from build123d import *

# Parameters (mm, degrees)
ESTRUSIONE_ESTRUSIONE1_DEPTH = 11
SCHIZZO4_R                   = 12
TAGLIO_ESTRUSIONE1_DEPTH     = 64.600314465
FORO_5_0_5_1_D               = 5
FORO_5_0_5_2_D               = 5
RACCORDO1_R                  = 0.2


with BuildPart() as part:
    # Schizzo2 → Estrusione-Estrusione1 (new body)
    with BuildSketch(Plane(origin=(0, 0, 0), x_dir=(1, 0, 0), z_dir=(0, 0, -1))):
        Polygon((-60, -8), (-60, 8), (-45, 8), (-45, 18), (45, 18), (45, 8), (60, 8), (60, -8), (45, -8), (45, -18), (-45, -18), (-45, -8), align=None)
    extrude(amount=-ESTRUSIONE_ESTRUSIONE1_DEPTH)

    # Schizzo4 → Taglio-Estrusione1 (cut, through all)
    with BuildSketch(Plane.XY.offset(11)):
        Circle(SCHIZZO4_R)
    extrude(amount=-TAGLIO_ESTRUSIONE1_DEPTH, mode=Mode.SUBTRACT)

    # Foro Ø5.0 (5)-1 (through all)
    with Locations(Plane(origin=(0, -18, 0), x_dir=(-1, 0, 0), z_dir=(0, -1, 0))):
        with Locations((0, -5.5)):
            Hole(FORO_5_0_5_1_D / 2)

    # Foro Ø5.0 (5)-2 (through all)
    with Locations(Plane.XY.offset(11)):
        with Locations((-52.5, 0), (52.5, 0)):
            Hole(FORO_5_0_5_2_D / 2)

    # Raccordo1
    raccordo1_edges = [part.edges().sort_by_distance(p)[0] for p in [
        (45, -8, 5.5),
        (45, 8, 5.5),
        (-45, 8, 5.5),
        (-45, -8, 5.5),
    ]]
    fillet(raccordo1_edges, radius=RACCORDO1_R)


solid = part.part
Source: CAD feature listing. Evaluate the final solid. Frame: model axes, mm. A direction names the side the tool comes from. Give positions to 0.01 mm unless a question says otherwise; leave off trailing zeros. Loops run counter-clockwise (first coordinate to the right, second up) from the corner with the lowest first, then second, coordinate; pieces in that order, holes last. Notation, with made-up numbers: (34, 10) -> (85, 10) arc R9 cw to (85, 24) -> close; hole circle Ø4 at (68.5, 21.25). An arc over 180 degrees is marked (long way). Use a Markdown table: item, result. Add a question column.
1) Reachability of faces 4 (the face through (-53, -8, 5)), 5 (the face through (-52, 8, 5)), 6 (the face through (53, 8, 5)), 7 (the face through (52, -8, 5)) from +Z, -Z, +X, -X, +Y, -Y: full face, straight path, thin tool, end or side. Return the list, or none.
2) Section query A-A, the plane y = 0. Return the cut outline in (x, z).
3) Section query B-B, the plane x = -52.5. Return the cut outline in (y, z), then the cut area to 3 significant figures.
4) Section query D-D, the plane x = 0. Return the cut outline in (y, z), then the cut area to 3 significant figures.
5) First-contact query: pin 1 (5 mm diameter, centred on y = -12, z = 8, fed in from +X); pin 2 (5 mm diameter, centred on y = 13, z = 4.5, fed in from -X); pin 3 (1 mm diameter, centred on x = -47.5, z = 2, fed in from -Y). Flat tips, straight axial feed; report the tip coordinate or a pass-through.
6) Line query: line 1 along Z through (x, y) = (0, 13.5); line 2 along Y through (x, z) = (0, 2.5); line 3 along Y through (x, z) = (-52.5, 7.25). Output: solid intervals per line, ascending. Write a range as [from, to].
7) Section query C-C, the plane z = 1.5. Return the cut outline in (x, y), then the cut area to 3 significant figures.
8) Pull-direction query (X, two-part tool) for faces 1 (the face through (50.19, -0.96, 5.42)), 2 (the face through (-45, 13, 5)), 3 (the face through (0.8, -12.3, 11)); classes: +X half, -X half, draft (parallel to the pull), parting line (faces both ways), or undercut.
Numbers:
| question | item | result |
|---|---|---|
| 1 | face 4 | +Z, -Z, -X, -Y |
| 1 | face 5 | +Z, -Z, -X, +Y |
| 1 | face 6 | +Z, -Z, +X, +Y |
| 1 | face 7 | +Z, -Z, +X, -Y |
| 2 | outline | (-60, 0) -> (-55, 0) -> (-55, 11) -> (-60, 11) -> close; (-50, 0) -> (-12, 0) -> (-12, 11) -> (-50, 11) -> close; (12, 0) -> (50, 0) -> (50, 11) -> (12, 11) -> close; (55, 0) -> (60, 0) -> (60, 11) -> (55, 11) -> close |
| 3 | outline | (-8, 0) -> (-2.5, 0) -> (-2.5, 11) -> (-8, 11) -> close; (2.5, 0) -> (8, 0) -> (8, 11) -> (2.5, 11) -> close |
| 3 | area | 121 mm2 |
| 4 | outline | (-18, 0) -> (-12, 0) -> (-12, 3) -> (-18, 3) -> close; (-18, 8) -> (-12, 8) -> (-12, 11) -> (-18, 11) -> close; (12, 0) -> (18, 0) -> (18, 3) -> (12, 3) -> close; (12, 8) -> (18, 8) -> (18, 11) -> (12, 11) -> close |
| 4 | area | 72.0 mm2 |
| 5 | pin 1 | stops at x = 45 |
| 5 | pin 2 | stops at x = -45 |
| 5 | pin 3 | stops at y = -8 |
| 6 | line 1 | z = [0, 3], [8, 11] |
| 6 | line 2 | y = [-18, -12], [12, 18] |
| 6 | line 3 | y = [-8, -2.5], [2.5, 8] |
| 7 | outline | (-60, -8) -> (-45.2, -8) arc R0.2 cw to (-45, -8.2) -> (-45, -18) -> (45, -18) -> (45, -8.2) arc R0.2 cw to (45.2, -8) -> (60, -8) -> (60, 8) -> (45.2, 8) arc R0.2 cw to (45, 8.2) -> (45, 18) -> (-45, 18) -> (-45, 8.2) arc R0.2 cw to (-45.2, 8) -> (-60, 8) -> close; hole circle Ø5 at (-52.5, 0); hole circle Ø24 at (0, 0); hole circle Ø5 at (52.5, 0) |
| 7 | area | 3,230 mm2 |
| 8 | face 1 | undercut |
| 8 | face 2 | -X half |
| 8 | face 3 | draft |
